Here's how the part is built. I have some questions about the finished solid (model axes, mm). Round coordinates to 2 decimals unless told otherwise and drop trailing zeros. Write each loop counter-clockwise with the first axis right and the second up, starting at its lowest first coordinate (ties: lowest second). Pieces come first, ordered by that corner, then holes. Notation, with made-up numbers: (38.5, 25.25) -> (48.5, 25.25) arc R30 cw to (48.5, 64.25) -> close; hole circle Ø4 at (-22.5, 17.25). An arc over 180 degrees is marked (long way). Answer as CSV lines item,"result".
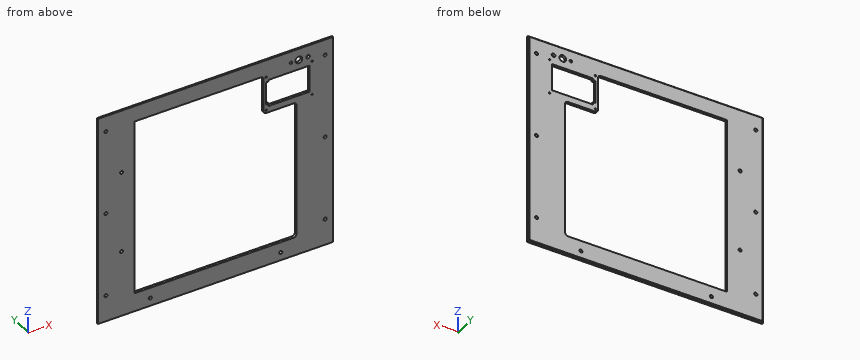
```python
from build123d import *

# Parameters (mm, degrees)
CROQUIS1_R              = 3
CROQUIS1_R_2            = 1.5
CROQUIS1_R_3            = 6.5
CROQUIS1_R_4            = 3.5
CROQUIS1_R_5            = 2.5
SALIENTE_EXTRUIR1_DEPTH = 5
CHAFL_N1_SIZE           = 2
REDONDEO1_R             = 5


with BuildPart() as part:
    # Croquis1 → Saliente-Extruir1 (new body)
    with BuildSketch(Plane(origin=(0, 0, 0), x_dir=(1, 0, 0), z_dir=(0, 1, 0))):
        Polygon((191.673151751, -229.571984436), (261.673151751, -229.571984436), (261.673151751, 170.428015564), (-188.326848249, 170.428015564), (-188.326848249, -229.571984436), (-118.326848249, -229.571984436), align=None)
        with Locations(Location((-173.326848249, 120.428015564, 0), (0, 0, 270))):
            Circle(CROQUIS1_R, mode=Mode.SUBTRACT)
        with Locations(Location((-173.326848249, -199.571984436, 0), (0, 0, 270))):
            Circle(CROQUIS1_R, mode=Mode.SUBTRACT)
        with Locations(Location((246.673151751, -199.571984436, 0), (0, 0, 270))):
            Circle(CROQUIS1_R, mode=Mode.SUBTRACT)
        with Locations(Location((246.673151751, 120.428015564, 0), (0, 0, 270))):
            Circle(CROQUIS1_R, mode=Mode.SUBTRACT)
        with Locations(Location((-173.326848249, -39.571984436, 0), (0, 0, 270))):
            Circle(CROQUIS1_R, mode=Mode.SUBTRACT)
        with Locations(Location((246.673151751, -39.571984436, 0), (0, 0, 270))):
            Circle(CROQUIS1_R, mode=Mode.SUBTRACT)
        with Locations(Location((-88.326848249, 155.428015564, 0), (0, 0, 270))):
            Circle(CROQUIS1_R, mode=Mode.SUBTRACT)
        with Locations(Location((161.673151751, 155.428015564, 0), (0, 0, 270))):
            Circle(CROQUIS1_R, mode=Mode.SUBTRACT)
        with Locations(Location((133.723151751, -131.571984436, 0), (0, 0, 270))):
            Circle(CROQUIS1_R_2, mode=Mode.SUBTRACT)
        with Locations(Location((133.723151751, -196.571984436, 0), (0, 0, 270))):
            Circle(CROQUIS1_R_2, mode=Mode.SUBTRACT)
        with Locations(Location((221.673151751, -196.571984436, 0), (0, 0, 270))):
            Circle(CROQUIS1_R_2, mode=Mode.SUBTRACT)
        with Locations(Location((221.673151751, -131.571984436, 0), (0, 0, 270))):
            Circle(CROQUIS1_R_2, mode=Mode.SUBTRACT)
        with Locations(Location((196.323151751, -207.921984436, 0), (0, 0, 270))):
            Circle(CROQUIS1_R_3, mode=Mode.SUBTRACT)
        with Locations(Location((214.073151751, -207.921984436, 0), (0, 0, 270))):
            Circle(CROQUIS1_R_4, mode=Mode.SUBTRACT)
        with Locations(Location((181.073151751, -207.921984436, 0), (0, 0, 270))):
            Circle(CROQUIS1_R_5, mode=Mode.SUBTRACT)
        with Locations(Location((-143.326848249, 45.178015564, 0), (0, 0, 270))):
            Circle(CROQUIS1_R, mode=Mode.SUBTRACT)
        with Locations(Location((-143.326848249, -109.321984436, 0), (0, 0, 270))):
            Circle(CROQUIS1_R, mode=Mode.SUBTRACT)
        Polygon((138.673151751, -186.171984436), (138.673151751, -189.571984436), (217.123151751, -189.571984436), (217.123151751, -138.571984436), (138.673151751, -138.571984436), (138.673151751, -143.171984436), (133.273151751, -143.171984436), (133.273151751, -186.171984436), align=None, mode=Mode.SUBTRACT)
        Polygon((-118.326848249, -199.571984436), (-118.326848249, 135.428015564), (191.673151751, 135.428015564), (191.673151751, -126.571984436), (128.723151751, -126.571984436), (128.723151751, -199.571984436), align=None, mode=Mode.SUBTRACT)
    extrude(amount=SALIENTE_EXTRUIR1_DEPTH)

    # Chaflán1
    chafl_n1_edges = [part.edges().sort_by_distance(p)[0] for p in [
        (261.673151751, 5, 29.571984436),
        (36.673151751, 5, -170.428015564),
        (-188.326848249, 5, 29.571984436),
        (36.673151751, 5, 229.571984436),
    ]]
    chamfer(chafl_n1_edges, length=CHAFL_N1_SIZE)

    # Redondeo1
    redondeo1_edges = [part.edges().sort_by_distance(p)[0] for p in [
        (191.673151751, 2.5, 126.571984436),
        (191.673151751, 2.5, -135.428015564),
        (128.723151751, 2.5, 199.571984436),
        (128.723151751, 2.5, 126.571984436),
    ]]
    fillet(redondeo1_edges, radius=REDONDEO1_R)


solid = part.part
```
1. Suppose I cut it at B-B on x = -43.5. Please give me the cut outline in (y, z), and give its area (3 significant figures).
Numbers:
outline,"(0, -170.43) -> (3, -170.43) -> (5, -168.43) -> (5, -135.43) -> (0, -135.43) -> close; (0, 199.57) -> (5, 199.57) -> (5, 227.57) -> (3, 229.57) -> (0, 229.57) -> close"
area,"321 mm^2"
2. Suppose I cut it at A-A on z = -16. Please give me the cut outline in (x, y).
Numbers:
outline,"(-188.33, 0) -> (-118.33, 0) -> (-118.33, 5) -> (-186.33, 5) -> (-188.33, 3) -> close; (191.67, 0) -> (261.67, 0) -> (261.67, 3) -> (259.67, 5) -> (191.67, 5) -> close"
3. If I drill on line 1 (X direction, y = 1.4, z = 171); line 2 (Z direction, x = 178.5, y = 2.15); line 3 (X direction, y = 4.35, z = 177), over which ranges is the centre line in solid material (lowest first)?
Numbers:
line 1,"x = -188.33 to -118.33, 128.72 to 133.27, 217.12 to 261.67"
line 2,"z = -170.43 to -135.43, 126.57 to 138.57, 189.57 to 229.57"
line 3,"x = -186.98 to -118.33, 128.72 to 133.27, 217.12 to 260.32"
4. Suppose I cut it at C-C on y = 4.2. Count the separate pieces of the cut face and the enclosed holes in it, and give its area (3 significant figures).
Numbers:
separate pieces,"1"
enclosed holes,"19"
area,"74,000 mm^2"
5. For pin 1 Ø3 at (x, z) = (181.07, 207.92) entering from -Y; pin 2 Ø9 at (x, z) = (214.07, 207.92) entering from -Y, each with a flat end and sliding along its axis, tell me the tip position at first contact or that it passes through.
Numbers:
pin 1,"passes through"
pin 2,"stops at y = 0"
